```python
from build123d import *

# Parameters (mm, degrees)
PIPE_TAP_DRILL_FOR_1_8_TAP1_D      = 8.4328
PIPE_TAP_DRILL_FOR_1_8_TAP1_DEPTH  = 15.246531286
PIPE_TAP_DRILL_FOR_1_8_TAP1_TIP    = 2.533468714
PIPE_TAP_DRILL_FOR_3_8_TAP2_D      = 14.2748
PIPE_TAP_DRILL_FOR_3_8_TAP2_DEPTH  = 12.7
PIPE_TAP_DRILL_FOR_3_8_TAP2_TIP    = 4.288582582
CIRPATTERN4_COUNT                  = 3
PIPE_TAP_DRILL_FOR_1_8_TAP2_D      = 8.4328
PIPE_TAP_DRILL_FOR_1_8_TAP2_DEPTH  = 10.166531286
PIPE_TAP_DRILL_FOR_1_8_TAP2_TIP    = 2.533468714
F_1_16_0_0625_DIAMETER_HOLE1_D     = 1.5875
F_1_16_0_0625_DIAMETER_HOLE1_DEPTH = 8.89
F_1_4_20_TAPPED_HOLE1_D            = 5.1054
F_1_4_20_TAPPED_HOLE1_DEPTH        = 11.166183098
F_1_4_20_TAPPED_HOLE1_TIP          = 1.533816902
F_29_0_136_DIAMETER_HOLE4_D        = 3.4544
F_29_0_136_DIAMETER_HOLE4_DEPTH    = 17.78
F_29_0_136_DIAMETER_HOLE4_TIP      = 1.037806461
CIRPATTERN3_COUNT                  = 3


with BuildPart() as part:
    # Sketch1 → Revolve1 (revolve)
    with BuildSketch(Plane.XY):
        Polygon((-31.75, 12.7), (-29.591, 12.7), (-29.591, 8.89), (-31.75, 8.89), (-31.75, 6.35), (-19.05, 6.35), (-19.05, 3.175), (-31.75, 3.175), (-31.75, 0.635), (-29.591, 0.635), (-29.591, -3.175), (-31.75, -3.175), (-31.75, -5.715), (-25.4, -5.715), (-25.4, 0), (0, 0), (0, 20.955), (-31.75, 20.955), (-31.75, 18.415), (-30.226, 18.415), (-30.226, 15.24), (-31.75, 15.24), align=None)
    revolve(axis=Axis((0, 26.246011395, 0), (0, -1, 0)))

    # Pipe Tap Drill for 1/8 Tap1
    with Locations(Plane(origin=(0, 20.955, 0), x_dir=(1, 0, 0), z_dir=(0, 1, 0))):
        with Locations((22.86, 0)):
            Hole(PIPE_TAP_DRILL_FOR_1_8_TAP1_D / 2, depth=PIPE_TAP_DRILL_FOR_1_8_TAP1_DEPTH)
            with Locations((0, 0, -(PIPE_TAP_DRILL_FOR_1_8_TAP1_DEPTH + PIPE_TAP_DRILL_FOR_1_8_TAP1_TIP / 2))):  # 118° drill point
                Cone(0, PIPE_TAP_DRILL_FOR_1_8_TAP1_D / 2, PIPE_TAP_DRILL_FOR_1_8_TAP1_TIP, mode=Mode.SUBTRACT)

    # Pipe Tap Drill for 3/8 Tap2
    with Locations(Plane(origin=(0, 20.955, 0), x_dir=(1, 0, 0), z_dir=(0, 1, 0))):
        with Locations((0, 0)):
            Hole(PIPE_TAP_DRILL_FOR_3_8_TAP2_D / 2, depth=PIPE_TAP_DRILL_FOR_3_8_TAP2_DEPTH)
            with Locations((0, 0, -(PIPE_TAP_DRILL_FOR_3_8_TAP2_DEPTH + PIPE_TAP_DRILL_FOR_3_8_TAP2_TIP / 2))):  # 118° drill point
                Cone(0, PIPE_TAP_DRILL_FOR_3_8_TAP2_D / 2, PIPE_TAP_DRILL_FOR_3_8_TAP2_TIP, mode=Mode.SUBTRACT)

    # Sketch7 → #39 (0.0995) Diameter Hole1 (revolve, cut)
    with BuildSketch(Plane(origin=(5.499261314, 0, 3.175), x_dir=(0, 0, -1), z_dir=(1, 0, 0))):
        Polygon((0, 0), (0, 11.176), (1.26365, 10.416722479), (1.26365, 0), align=None)
    f_39_0_0995_diameter_hole1 = revolve(axis=Axis((5.499261314, -6.35, 3.175), (0, 1, 0)), mode=Mode.SUBTRACT)

    # CirPattern4: #39 (0.0995) Diameter Hole1 ×3 about axis
    cirpattern4_axis = Axis((0, 0, 0), (0, 1, 0))
    for i in range(1, CIRPATTERN4_COUNT):
        add(f_39_0_0995_diameter_hole1.rotate(cirpattern4_axis, i * 360 / CIRPATTERN4_COUNT), mode=Mode.SUBTRACT)

    # Pipe Tap Drill for 1/8 Tap2
    with Locations(Plane(origin=(0, 20.955, 0), x_dir=(1, 0, 0), z_dir=(0, 1, 0))):
        with Locations((-17.78, 0)):
            Hole(PIPE_TAP_DRILL_FOR_1_8_TAP2_D / 2, depth=PIPE_TAP_DRILL_FOR_1_8_TAP2_DEPTH)
            with Locations((0, 0, -(PIPE_TAP_DRILL_FOR_1_8_TAP2_DEPTH + PIPE_TAP_DRILL_FOR_1_8_TAP2_TIP / 2))):  # 118° drill point
                Cone(0, PIPE_TAP_DRILL_FOR_1_8_TAP2_D / 2, PIPE_TAP_DRILL_FOR_1_8_TAP2_TIP, mode=Mode.SUBTRACT)

    # 1/16 (0.0625) Diameter Hole1
    with Locations(Plane(origin=(0, -5.715, 0), x_dir=(-1, 0, 0), z_dir=(0, -1, 0))):
        with Locations((-17.597636205, -10.16)):
            f_1_16_0_0625_diameter_hole1 = Hole(F_1_16_0_0625_DIAMETER_HOLE1_D / 2, depth=F_1_16_0_0625_DIAMETER_HOLE1_DEPTH)

    # 1/4-20 Tapped Hole1
    with Locations(Plane(origin=(0, 0, 0), x_dir=(-1, 0, 0), z_dir=(0, -1, 0))):
        with Locations((0, 0)):
            Hole(F_1_4_20_TAPPED_HOLE1_D / 2, depth=F_1_4_20_TAPPED_HOLE1_DEPTH)
            with Locations((0, 0, -(F_1_4_20_TAPPED_HOLE1_DEPTH + F_1_4_20_TAPPED_HOLE1_TIP / 2))):  # 118° drill point
                Cone(0, F_1_4_20_TAPPED_HOLE1_D / 2, F_1_4_20_TAPPED_HOLE1_TIP, mode=Mode.SUBTRACT)

    # #29 (0.136) Diameter Hole4
    with Locations(Plane(origin=(0, -5.715, 0), x_dir=(-1, 0, 0), z_dir=(0, -1, 0))):
        with Locations((15.24, 0)):
            Hole(F_29_0_136_DIAMETER_HOLE4_D / 2, depth=F_29_0_136_DIAMETER_HOLE4_DEPTH)
            with Locations((0, 0, -(F_29_0_136_DIAMETER_HOLE4_DEPTH + F_29_0_136_DIAMETER_HOLE4_TIP / 2))):  # 118° drill point
                Cone(0, F_29_0_136_DIAMETER_HOLE4_D / 2, F_29_0_136_DIAMETER_HOLE4_TIP, mode=Mode.SUBTRACT)

    # CirPattern3: 1/16 (0.0625) Diameter Hole1 ×3 about axis
    cirpattern3_axis = Axis((0, 0, 0), (0, 1, 0))
    for i in range(1, CIRPATTERN3_COUNT):
        add(f_1_16_0_0625_diameter_hole1.rotate(cirpattern3_axis, i * 360 / CIRPATTERN3_COUNT), mode=Mode.SUBTRACT)


solid = part.part
```
Geometry: final body of the model. Coordinates: model frame, mm. A direction names the side the tool comes from. Coordinates: 2 decimals unless noted, no trailing zeros. Order: outer loops, then holes, each group sorted by start corner. A loop starts at its lowest first (then second) coordinate and runs counter-clockwise, first axis right, second up.
Item 1: Draft query along Z for faces 4 (the face through (-6.752, 3.978, 3.34)), 5 (the face through (6.41, 10.77, 28.89)), 6 (the face through (-9.3, 0.635, -28.4)). Return one class per face: released by +Z, released by -Z, zero draft, split by the parting line, or undercut.
Answer:
face 4: undercut
face 5: split by the parting line
face 6: zero draft
Item 2: Material intervals for line 1 along Y through (x, z) = (19, 21) (3 decimals); line 2 along Y through (x, z) = (3, 23.5) (3 decimals); line 3 along X through (y, z) = (-1.55, 0), sorted ascending.
Answer:
line 1: y = -5.715 to 3.175, 6.35 to 20.955
line 2: y = 0 to 3.175, 6.35 to 20.955
line 3: x = -29.59 to -25.4, 25.4 to 29.59
Item 3: Access query for faces 1 (the face through (9.3, 8.89, -28.4)), 2 (the face through (-3.837, 14.516, -6.018)), 3 (the face through (0, 0, 5)). Directions: +Z, -Z, +X, -X, +Y, -Y. A direction counts if a zero-diameter tool reaches every point of the face in a straight line with its end or side. Return the directions, or none.
Answer:
face 1: none
face 2: +Y
face 3: -Y
Item 4: Contact query for flat-ended pins moving along their axis: P1, Ø6.5, axis at x = -17.78, z = 0, coming from the -Y side; P2, Ø2, axis at x = -11.5, y = -2, coming from the +Z side; P3, Ø3, axis at y = 6.5, z = 5.5, coming from the -X side; P4, Ø19, axis at x = 2.5, z = -0.5, coming from the +Y side (3 decimals). Output: stop coordinate, or through.
Answer:
P1: stops at y = 0
P2: stops at z = 27.67
P3: stops at x = -31.5
P4: stops at y = 20.955
Item 5: Section query B-B (y = 17.5). Output: boundary loops of the cut face in (x, z), then the cut area to 3 significant figures.
Answer:
outline: circle Ø60.45 at (0, 0); hole circle Ø8.43 at (-17.78, 0); hole circle Ø14.27 at (0, 0); hole circle Ø8.43 at (22.86, 0)
area: 2,600 mm2
Item 6: Section query A-A (y = 2). State how many separate pieces and enclosed holes the cut face has, then the cut area to 3 significant figures.
Answer:
separate pieces: 1
enclosed holes: 8
area: 3,120 mm2
